from build123d import *

# Parameters (mm, degrees)
PAD001_DEPTH         = 3
SKETCH024_R          = 1.2
POCKET008_DEPTH      = 3.001
PAD002_DEPTH         = 1
SKETCH023_R          = 1.2
POCKET010_DEPTH      = 4.001
POCKET010_DEPTH_BACK = 0.001
POCKET011_DEPTH      = 1.75


with BuildPart() as part:
    # Sketch022 → Pad001 (new body)
    with BuildSketch(Plane.XY):
        with BuildLine():
            Line((-6.5, 0), (6.5, 0))
            ThreePointArc((6.5, 0), (7.914214, 0.585786), (8.5, 2))
            Line((8.5, 2), (8.5, 25))
            ThreePointArc((8.5, 25), (7.914214, 26.414214), (6.5, 27))
            Line((6.5, 27), (-6.5, 27))
            ThreePointArc((-6.5, 27), (-7.914214, 26.414214), (-8.5, 25))
            Line((-8.5, 25), (-8.5, 2))
            ThreePointArc((-8.5, 2), (-7.914214, 0.585786), (-6.5, 0))
        make_face()
    extrude(amount=-PAD001_DEPTH)

    # Sketch024 → Pocket008 (cut, through all)
    with BuildSketch(Plane.XY):
        with Locations((-5.5, 24)):
            Circle(SKETCH024_R)
        with Locations((5.5, 24)):
            Circle(SKETCH024_R)
        with Locations((5.5, 3)):
            Circle(SKETCH024_R)
        with Locations((-5.5, 3)):
            Circle(SKETCH024_R)
    extrude(amount=-POCKET008_DEPTH, mode=Mode.SUBTRACT)

    # Sketch026 (on DatumPlane) → Pad002 (join)
    with BuildSketch(Plane.XY.offset(-3)):
        with BuildLine():
            ThreePointArc((-3.711996, 20.131824), (-7.6, 13.5), (-3.711996, 6.868176))
            ThreePointArc((-2.735155, 5.550893), (-3.08235, 6.314261), (-3.711996, 6.868176))
            ThreePointArc((-2.735155, 5.550893), (0, 3.35), (2.735155, 5.550893))
            ThreePointArc((3.711996, 6.868176), (3.08235, 6.314261), (2.735155, 5.550893))
            ThreePointArc((3.711996, 6.868176), (7.6, 13.5), (3.711996, 20.131824))
            ThreePointArc((2.735155, 21.449107), (3.08235, 20.685739), (3.711996, 20.131824))
            ThreePointArc((2.735155, 21.449107), (0, 23.65), (-2.735155, 21.449107))
            ThreePointArc((-3.711996, 20.131824), (-3.08235, 20.685739), (-2.735155, 21.449107))
        make_face()
    extrude(amount=-PAD002_DEPTH)

    # Sketch023 → Pocket010 (cut, two sides)
    with BuildSketch(Plane.XY) as pocket010_sk:
        with Locations((0, 6.15)):
            Circle(SKETCH023_R)
        with Locations((0, 20.85)):
            Circle(SKETCH023_R)
    extrude(amount=-POCKET010_DEPTH, mode=Mode.SUBTRACT)
    extrude(pocket010_sk.sketch, amount=POCKET010_DEPTH_BACK, mode=Mode.SUBTRACT)

    # Sketch027 → Pocket011 (cut)
    with BuildSketch(Plane.XY):
        Polygon((4.287564, 0.9), (6.712436, 0.9), (7.924871, 3), (6.712436, 5.1), (4.287564, 5.1), (3.075129, 3), align=None)
        Polygon((6.712436, 26.1), (4.287564, 26.1), (3.075129, 24), (4.287564, 21.9), (6.712436, 21.9), (7.924871, 24), align=None)
        Polygon((-4.287564, 21.9), (-3.075129, 24), (-4.287564, 26.1), (-6.712436, 26.1), (-7.924871, 24), (-6.712436, 21.9), align=None)
        Polygon((-4.287564, 0.9), (-3.075129, 3), (-4.287564, 5.1), (-6.712436, 5.1), (-7.924871, 3), (-6.712436, 0.9), align=None)
    extrude(amount=-POCKET011_DEPTH, mode=Mode.SUBTRACT)


solid = part.part
Design review of the part built by this model. Coordinates are the model's own, in mm. A direction names the side the tool comes from. Coordinates: 2 decimals unless noted, no trailing zeros. Write each loop counter-clockwise with the first axis right and the second up, starting at its lowest first coordinate (ties: lowest second). Pieces come first, ordered by that corner, then holes. Notation, with made-up numbers: (-33, -3) -> (-7, -3) arc R27 ccw to (-7, 33) -> close; hole circle Ø11 at (22.5, 39). An arc over 180 degrees is marked (long way). Write each question's results on one line, items separated by ' | '. Start each with the question number.
(1) Take a section at D-D on x = -5.5. Write out the cut boundary in (y, z) (3 decimals), and give its area (3 significant figures).
(2) The part is to be moulded in two halves that separate along X. For faces 5 (the face through (7.9, 0.57, -1.48)), 6 (the face through (-6, 0.9, -1)), 7 (the face through (-8.5, 14, -1)), say which applies: pulls with the +X half, pulls with the -X half, needs draft (parallel to the pull), parting line crosses it, or undercut.
(3) Tool access review of faces 1 (the face through (3.69, 4.065, -0.863)), 2 (the face through (-0.05, 3.35, -3.49)), 3 (the face through (-3.089, 20.676, -3.493)), 4 (the face through (7.6, 13.4, -3.5)): name each direction out of +Z, -Z, +X, -X, +Y, -Y from which nothing blocks a thin tool from reaching the whole face with its end or side.
(4) Take a section at B-B on z = -0.95. Give the number of separate pieces and of enclosed holes in the cut face, and give its area (3 significant figures).
(5) Clearance check with flat-ended pins moving along their axes: P1, Ø1.4, axis at x = -5.5, y = 24, coming from the +Z side; P2, Ø4, axis at x = 5.5, y = 24, coming from the +Z side. State where each tip first meets the part, or that it passes through.
(6) Take a section at A-A on z = -3.4. Write out the cut boundary in (x, y), and give its area (3 significant figures).
(7) For line 1 along Y through (x, z) = (5.5, -2.05); line 2 along Y through (x, z) = (3.5, -0.5); line 3 along X through (y, z) = (23.75, -2.8), list the stretches that pass through material, from the lowest coordinate up. Write a range as from..to.
(8) Take a section at C-C on y = 6.15. Write out the cut boundary in (x, z), and give its area (3 significant figures).
Results found:
1) outline: (0, -3) -> (1.8, -3) -> (1.8, -1.75) -> (0.9, -1.75) -> (0.9, 0) -> (0, 0) -> close; (4.2, -3) -> (8.255, -3) -> (8.255, -4) -> (18.745, -4) -> (18.745, -3) -> (22.8, -3) -> (22.8, -1.75) -> (21.9, -1.75) -> (21.9, 0) -> (5.1, 0) -> (5.1, -1.75) -> (4.2, -1.75) -> close; (25.2, -3) -> (27, -3) -> (27, 0) -> (26.1, 0) -> (26.1, -1.75) -> (25.2, -1.75) -> close | area: 70.8 mm2
2) face 5: pulls with the +X half | face 6: undercut | face 7: pulls with the -X half
3) face 1: +Z | face 2: -Z, -Y | face 3: -Z, -X, +Y | face 4: -Z, +X
4) separate pieces: 1 | enclosed holes: 6 | area: 385 mm2
5) P1: passes through | P2: stops at z = -1.75
6) outline: (-3.71, 6.87) arc R2 cw to (-2.74, 5.55) arc R2.8 ccw to (2.74, 5.55) arc R2 cw to (3.71, 6.87) arc R7.6 ccw to (3.71, 20.13) arc R2 cw to (2.74, 21.45) arc R2.8 ccw to (-2.74, 21.45) arc R2 cw to (-3.71, 20.13) arc R7.6 ccw to start; hole circle Ø2.4 at (0, 6.15); hole circle Ø2.4 at (0, 20.85) | area: 197 mm2
7) line 1: y = 0..1.8, 4.2..22.8, 25.2..27 | line 2: y = 0..2.26, 3.74..23.26, 24.74..27 | line 3: x = -8.5..-6.67, -4.33..4.33, 6.67..8.5
8) outline: (-8.5, -3) -> (-2.97, -3) -> (-2.97, -4) -> (-1.2, -4) -> (-1.2, 0) -> (-8.5, 0) -> close; (1.2, -4) -> (2.97, -4) -> (2.97, -3) -> (8.5, -3) -> (8.5, 0) -> (1.2, 0) -> close | area: 47.3 mm2
